Source: three-view drawing plus pictorial views. Frame: mm from the lowest corner of the part. Give positions to 0.01 mm unless a question says otherwise; leave off trailing zeros. Loops run counter-clockwise (first coordinate to the right, second up) from the corner with the lowest first, then second, coordinate; pieces in that order, holes last. Notation, with made-up numbers: (-15, -7) - (4, -7) arc R18 ccw to (4, 18) - close; hole circle Ø1 at (28, 28). An arc over 180 degrees is marked (long way). Put each result on its own line as item: value.
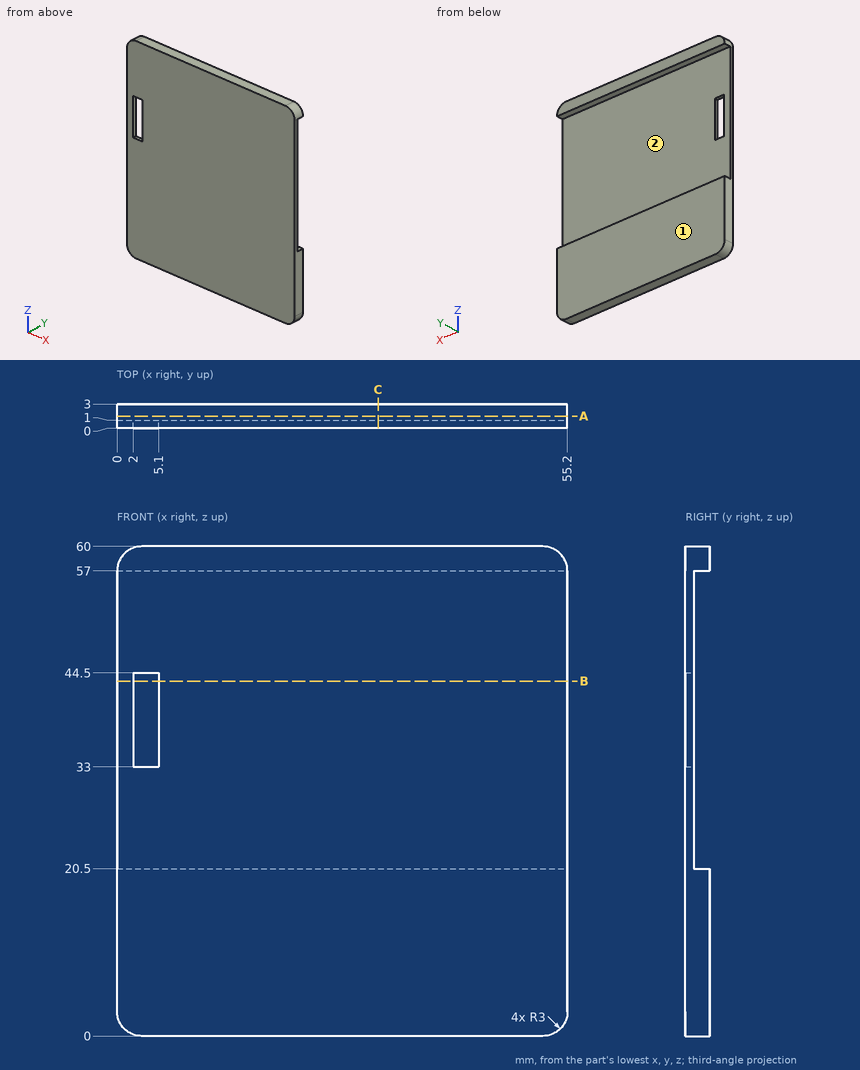
1) Section query B-B, the plane z = 43.5. Output: boundary loops of the cut face in (x, y).
Check result:
outline: (0, 0) - (2, 0) - (2, 1) - (0, 1) - close; (5.1, 0) - (55.2, 0) - (55.2, 1) - (5.1, 1) - close
2) Pin query (flat end, axial travel): P1, Ø18, axis at x = 29.5, z = 44.5, coming from the +Y side; P2, Ø1.5, axis at y = 2.5, z = 29, coming from the +X side. Return the tip coordinate at first contact, or that it passes through.
Check result:
P1: y = 1
P2: through
3) Section query A-A, the plane y = 1.5. Output: boundary loops of the cut face in (x, z).
Check result:
outline: (0, 3) arc R3 ccw to (3, 0) - (52.2, 0) arc R3 ccw to (55.2, 3) - (55.2, 20.5) - (0, 20.5) - close; (0, 57) - (55.2, 57) arc R3 ccw to (52.2, 60) - (3, 60) arc R3 ccw to start
4) Section query C-C, the plane x = 32. Output: boundary loops of the cut face in (y, z), plus the area to 3 significant figures.
Check result:
outline: (0, 0) - (3, 0) - (3, 20.5) - (1, 20.5) - (1, 57) - (3, 57) - (3, 60) - (0, 60) - close
area: 107 mm²
5) Mould query, pull axis Z, two halves, no side actions, for the marked faces 1 and 2. Classes: pulls with the +Z half, pulls with the -Z half, needs draft (parallel to the pull), parting line crosses it, or undercut.
Check result:
face 1: needs draft
face 2: undercut
6) Material intervals for line 1 along X through (y, z) = (0.3, 34.5); line 2 along Z through (x, y) = (42, 1.1); line 3 along Y through (x, z) = (23, 51), sorted ascending. Write a range as [from, to].
Check result:
line 1: [0, 2], [5.1, 55.2]
line 2: [0, 20.5], [57, 60]
line 3: [0, 1]
